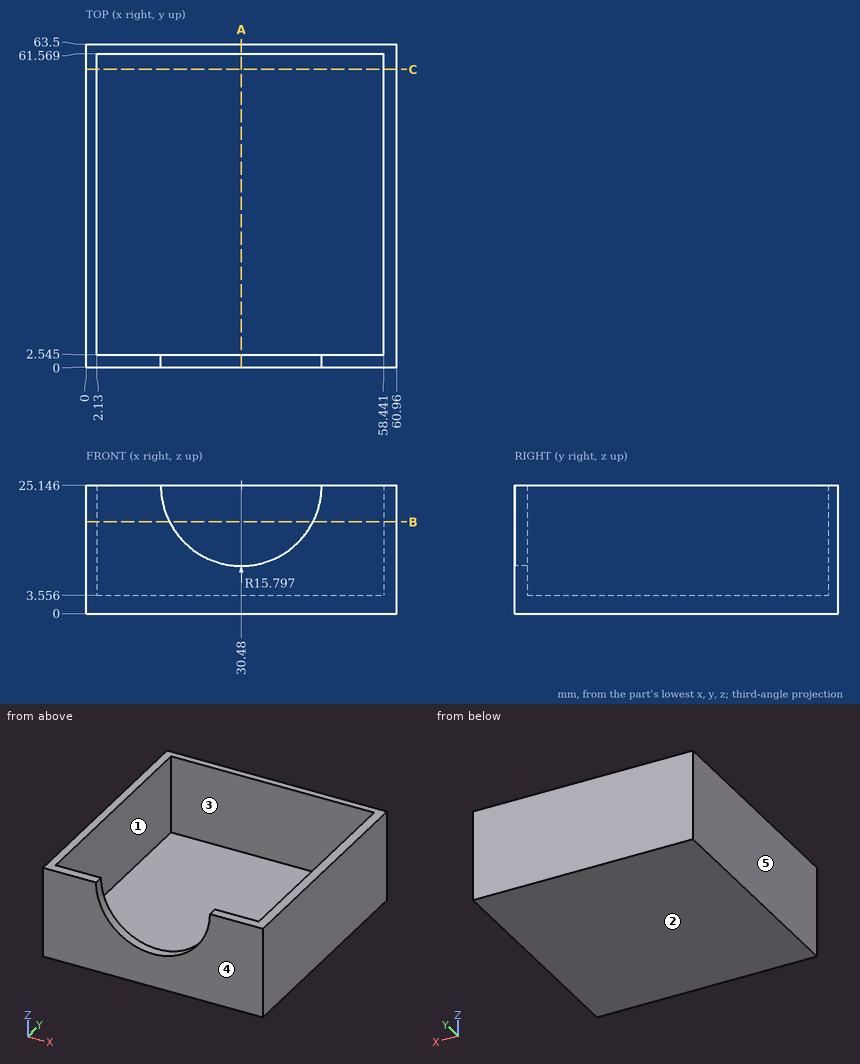
Could you check a few things on this drawing? It's one solid part, dimensions in mm from its lowest x, y, z. A direction names the side the tool comes from. Coordinates: 2 decimals unless noted, no trailing zeros. Write each loop counter-clockwise with the first axis right and the second up, starting at its lowest first coordinate (ties: lowest second). Pieces come first, ordered by that corner, then holes. Notation, with made-up numbers: (-15.5, 84.25) - (34.5, 84.25) arc R24 ccw to (34.5, 104.25) - close; hole circle Ø8 at (-39.5, -16.75). An arc over 180 degrees is marked (long way). Write item = value, one per line.
1) Will these pins go through, and if not, where does the flat tip stop? pin 1 Ø8 at (x, z) = (14, 6) entering from -Y; pin 2 Ø4 at (x, y) = (11.5, 27) entering from +Z; pin 3 Ø6.5 at (x, z) = (30, 14) entering from -Y.
Result set:
pin_1 = 0
pin_2 = 3.56
pin_3 = 61.57
2) Suppose I cut it at C-C on y = 58.5. Please give me the cut outline in (x, z).
Result set:
outline = (0, 0) - (60.96, 0) - (60.96, 25.15) - (58.44, 25.15) - (58.44, 3.56) - (2.13, 3.56) - (2.13, 25.15) - (0, 25.15) - close
3) We'd pull the mould along Y, two halves only. Please class the marked faces 3, 4 and 5: +Y half, -Y half, draft (parallel to the pull), parting line (faces both ways), or undercut.
Result set:
face_3 = undercut
face_4 = -Y half
face_5 = draft
4) Please list where these lines run through material, in increasing order: line 1 (Y direction, x = 9, z = 16) (1 decimal); line 2 (X direction, y = 21.5, z = 23.5); line 3 (Y direction, x = 32.5, z = 23.5). Write a range as [from, to].
Result set:
line_1 = [0, 2.5], [61.6, 63.5]
line_2 = [0, 2.13], [58.44, 60.96]
line_3 = [61.57, 63.5]
5) For the marked faces 1 and 2, which set-ups out of +Z, -Z, +X, -X, +Y, -Y let a thin tool reach every point of the face, with its end or its side?
Result set:
face_1 = +Z
face_2 = -Z, +X, -X, +Y, -Y
6) Suppose I cut it at A-A on x = 30.48. Please give me the cut outline in (y, z) (1 decimal), plus the area to 3 significant figures.
Result set:
outline = (0, 0) - (63.5, 0) - (63.5, 25.1) - (61.6, 25.1) - (61.6, 3.6) - (2.5, 3.6) - (2.5, 9.3) - (0, 9.3) - close
area = 282 mm2
7) Suppose I cut it at B-B on z = 18. Please give me the cut outline in (x, y) (1 decimal).
Result set:
outline = (0, 0) - (16.4, 0) - (16.4, 2.5) - (2.1, 2.5) - (2.1, 61.6) - (58.4, 61.6) - (58.4, 2.5) - (44.6, 2.5) - (44.6, 0) - (61, 0) - (61, 63.5) - (0, 63.5) - close
